Source: CAD feature listing. Evaluate the final solid. Frame: model axes, mm. Give positions to 0.01 mm unless a question says otherwise; leave off trailing zeros. Loops run counter-clockwise (first coordinate to the right, second up) from the corner with the lowest first, then second, coordinate; pieces in that order, holes last. Notation, with made-up numbers: (10, 25.25) -> (29, 25.25) arc R26 cw to (29, 54.25) -> close; hole circle Ø1 at (-7.5, 11.5). An arc over 180 degrees is marked (long way). Return JSON: item names as keys, results as strings. Group by question number.
(1) Ray query, line 1 (Y direction, x = 0.1, z = 3.75); line 2 (X direction, y = 0.9, z = 2.75). Return the intervals inside material, ascending. Write a range as from..to.
(2) Cut plane B-B on z = 18. Return loops of the section in (x, y), then the cut area to 3 significant figures.
(3) Cut plane A-A on z = 2.25. Return loops of the section in (x, y).
(4) Pin query (flat end, axial travel): pin 1 (0.7 mm diameter, centred on x = -0.5, z = 3, fed in from -Y) (3 decimals); pin 2 (1 mm diameter, centred on y = -1.5, z = 14, fed in from +X); pin 3 (1.5 mm diameter, centred on x = -1.5, y = 1.5, fed in from +Z). Return the tip coordinate at first contact, or that it passes through.
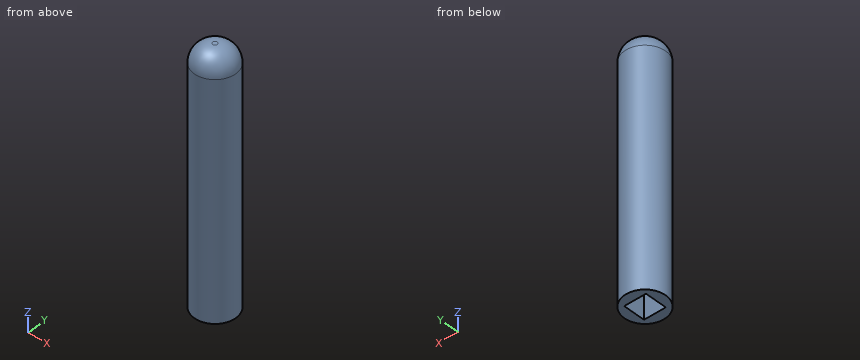
```python
from build123d import *

# Parameters (mm, degrees)
SKETCH_1_R          = 2.25
EXTRUDE_2_DEPTH     = 27.5
SKETCH_7_W          = 2.4
SKETCH_7_H          = 2.4
CUT_EXTRUDE_3_DEPTH = 4.5
FILLET_2_R          = 2


with BuildPart() as part:
    # 草图1 → 凸台-拉伸2 (new body)
    with BuildSketch(Plane.XY):
        Circle(SKETCH_1_R)
    extrude(amount=EXTRUDE_2_DEPTH)

    # 草图7 → 切除-拉伸3 (cut)
    with BuildSketch(Plane.XY):
        Rectangle(SKETCH_7_W, SKETCH_7_H)
    extrude(amount=CUT_EXTRUDE_3_DEPTH, mode=Mode.SUBTRACT)

    # 圆角2
    fillet_2_edges = [part.edges().sort_by_distance(p)[0] for p in [
        (-2.25, 0, 27.5),
    ]]
    fillet(fillet_2_edges, radius=FILLET_2_R)


solid = part.part
```
Answers:
{
 "1": {"line 1": "-2.25..-1.2, 1.2..2.25", "line 2": "-2.06..-1.2, 1.2..2.06"},
 "2": {"outline": "circle Ø4.5 at (0, 0)", "area": "15.9 mm²"},
 "3": {"outline": "circle Ø4.5 at (0, 0); hole (-1.2, -1.2) -> (1.2, -1.2) -> (1.2, 1.2) -> (-1.2, 1.2) -> close"},
 "4": {"pin 1": "y = -2.245", "pin 2": "x = 2.02", "pin 3": "z = 27.16"}
}
